```python
from build123d import *

# Parameters (mm, degrees)
F0_R     = 0.75
F1_DEPTH = 5
F2_R     = 1.575
F3_DEPTH = 5.001
F4_R     = 4.5
F5_DEPTH = 3
F6_R     = 2
F7_DEPTH = 2
F8_W     = 43.103866
F8_H     = 7.897038
F9_DEPTH = 16.001


with BuildPart() as f1:
    # F0 (on Top) → F1 (new body)
    with BuildSketch(Plane.XY):
        with BuildLine():
            Line((-8, 35), (-8, 0))
            Line((-8, 0), (-8, -35))
            ThreePointArc((-8, -35), (0, -43), (8, -35))
            Line((8, -35), (8, 0))
            Line((8, 0), (8, 35))
            ThreePointArc((8, 35), (0, 43), (-8, 35))
        make_face()
        with Locations((-2.969848, -37.969848)):
            Circle(F0_R, mode=Mode.SUBTRACT)
        with Locations((-2.969848, -32.030152)):
            Circle(F0_R, mode=Mode.SUBTRACT)
        with Locations((2.969848, -37.969848)):
            Circle(F0_R, mode=Mode.SUBTRACT)
        with Locations((2.969848, -32.030152)):
            Circle(F0_R, mode=Mode.SUBTRACT)
        with Locations((-2.969848, 32.030152)):
            Circle(F0_R, mode=Mode.SUBTRACT)
        with Locations((-2.969848, 37.969848)):
            Circle(F0_R, mode=Mode.SUBTRACT)
        with Locations((2.969848, 32.030152)):
            Circle(F0_R, mode=Mode.SUBTRACT)
        with Locations((2.969848, 37.969848)):
            Circle(F0_R, mode=Mode.SUBTRACT)
    extrude(amount=F1_DEPTH)

    # F2 (on face) → F3 (cut, through all)
    with BuildSketch(Plane.XY.offset(5)):
        with Locations((0, 5)):
            Circle(F2_R)
        with Locations((0, -5)):
            Circle(F2_R)
    extrude(amount=-F3_DEPTH, mode=Mode.SUBTRACT)

    # F4 (on face) → F5 (cut)
    with BuildSketch(Plane.XY.offset(5)):
        with Locations((0, 5)):
            Circle(F4_R)
        with Locations((0, -5)):
            Circle(F4_R)
    extrude(amount=-F5_DEPTH, mode=Mode.SUBTRACT)

    # F6 (on face) → F7 (cut)
    with BuildSketch(Plane(origin=(0, 0, 0), x_dir=(1, 0, 0), z_dir=(0, 0, -1))):
        with Locations((-2.969848, 37.969848)):
            Circle(F6_R)
        with Locations((2.969848, 37.969848)):
            Circle(F6_R)
        with Locations((2.969848, 32.030152)):
            Circle(F6_R)
        with Locations((-2.969848, 32.030152)):
            Circle(F6_R)
        with Locations((-2.969848, -32.030152)):
            Circle(F6_R)
        with Locations((-2.969848, -37.969848)):
            Circle(F6_R)
        with Locations((2.969848, -37.969848)):
            Circle(F6_R)
        with Locations((2.969848, -32.030152)):
            Circle(F6_R)
    extrude(amount=-F7_DEPTH, mode=Mode.SUBTRACT)

    # F8 (on face) → F9 (cut, through all)
    with BuildSketch(Plane.YZ.offset(8)):
        with Locations((-31.750295, 3.948519)):
            Rectangle(F8_W, F8_H)
    extrude(amount=-F9_DEPTH, mode=Mode.SUBTRACT)


solid = f1.part
```
Here's how the part is built. I have some questions about the finished solid (model axes, mm). A direction names the side the tool comes from. Round coordinates to 2 decimals unless told otherwise and drop trailing zeros. Order: outer loops, then holes, each group sorted by start corner. A loop starts at its lowest first (then second) coordinate and runs counter-clockwise, first axis right, second up. Notation, with made-up numbers: M 76.25,-28 L 103.25,-28 A25 cw 103.25,3 Z; hole C 32,53.5 d7. An arc over 180 degrees is marked long. Answer as CSV lines item,"result".
Item 1: Imagine slicing it at C-C on z = 3.9. List the corners of the cut face in (x, y) for me.
From the geometry:
outline,"M -8,-10.2 L 8,-10.2 L 8,35 A8 ccw -8,35 Z; hole C 0,-5 d9; hole C 0,5 d9; hole C -2.97,32.03 d1.5; hole C -2.97,37.97 d1.5; hole C 2.97,32.03 d1.5; hole C 2.97,37.97 d1.5"
Item 2: We'd pull the mould along X, two halves only. Please class faces 1 (the cylindrical face through (-3.067, 32.774, 3.479)), 2 (the flat face through (0, 17, 5)), 3 (the cylindrical face through (0, 43, 2)): +X half, -X half, draft (parallel to the pull), parting line (faces both ways), or undercut.
From the geometry:
face 1,"undercut"
face 2,"draft"
face 3,"parting line"
Item 3: Which directions (+Z, -Z, +X, -X, +Y, -Y) give clear straight access to the entire face, cutting with the end or side of a thin tool? Please do faces 4 (the cylindrical face through (-2.047, 39.744, 0.986)), 5 (the flat face through (8, 12, 2)), 6 (the flat face through (0, -7, 2)).
From the geometry:
face 4,"-Z"
face 5,"+Z, -Z, +X, +Y, -Y"
face 6,"+Z"
Item 4: Imagine slicing it at A-A on x = 0. List the corners of the cut face in (y, z) for me (3 decimals).
From the geometry:
outline,"M -10.198,0 L -6.575,0 L -6.575,2 L -9.5,2 L -9.5,5 L -10.198,5 Z; M -3.425,0 L 3.425,0 L 3.425,2 L 0.5,2 L 0.5,5 L -0.5,5 L -0.5,2 L -3.425,2 Z; M 6.575,0 L 43,0 L 43,5 L 9.5,5 L 9.5,2 L 6.575,2 Z"
Item 5: Imagine slicing it at D-D on y = 4. List the corners of the cut face in (x, z) for me.
From the geometry:
outline,"M -8,0 L -1.22,0 L -1.22,2 L -4.39,2 L -4.39,5 L -8,5 Z; M 1.22,0 L 8,0 L 8,5 L 4.39,5 L 4.39,2 L 1.22,2 Z"
Item 6: For pin 1 (2.5 mm diameter, centred on x = -2.97, y = 32.03, fed in from -Z); pin 2 (3 mm diameter, centred on x = 6.5, z = 2.5, fed in from +Y) (3 decimals); pin 3 (8 mm diameter, centred on x = 0, y = -5, fed in from +Z); pin 4 (1.4 mm diameter, centred on x = -2.97, y = 32.03, fed in from +Z), each with a flat end and sliding along its axis, tell me the tip position at first contact or that it passes through.
From the geometry:
pin 1,"z = 2"
pin 2,"y = 41.245"
pin 3,"z = 2"
pin 4,"through"
Item 7: Please list where these lines run through material, in increasing order: L1, parallel to Y at x = 0, z = 0.45 (3 decimals); L2, parallel to Y at x = 1.5, z = 4.3; L3, parallel to Z at x = -2.75, y = 4.5. Write a range as [from, to].
From the geometry:
L1,"[-10.198, -6.575], [-3.425, 3.425], [6.575, 43]"
L2,"[-10.2, -9.24], [-0.76, 0.76], [9.24, 42.86]"
L3,"[0, 2]"
Item 8: Imagine slicing it at B-B on y = -5. List the corners of the cut face in (x, z) for me (3 decimals), and give its area (3 significant figures).
From the geometry:
outline,"M -8,0 L -1.575,0 L -1.575,2 L -4.5,2 L -4.5,5 L -8,5 Z; M 1.575,0 L 8,0 L 8,5 L 4.5,5 L 4.5,2 L 1.575,2 Z"
area,"46.7 mm2"
